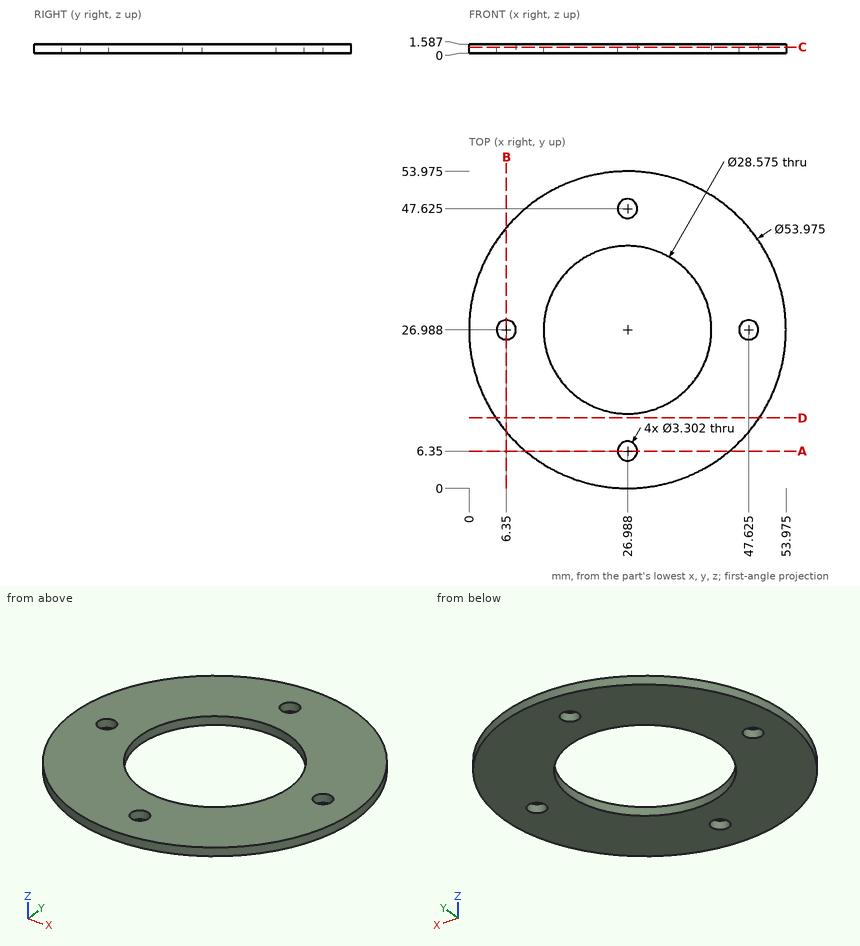
Job drawing, mm, ordinate dimensions from the low corner. One solid piece. Give positions to 0.01 mm unless a question says otherwise; leave off trailing zeros. Order: outer loops, then holes, each group sorted by start corner. A loop starts at its lowest first (then second) coordinate and runs counter-clockwise, first axis right, second up. Notation, with made-up numbers: (8.5, 80) - (62.5, 80) arc R26 ccw to (62.5, 116) - close; hole circle Ø9 at (56, 87.25). An arc over 180 degrees is marked (long way). Answer in a Markdown table with one row per item.
1. Saw through at C-C, the plane z = 1.05. Count the separate pieces of the cut face and the enclosed holes in it, plus the area to 3 significant figures.
Data:
| item | result |
|---|---|
| separate pieces | 1 |
| enclosed holes | 5 |
| area | 1,610 mm² |
2. Saw through at A-A, the plane y = 6.35. Give the cut face in (x, z).
Data:
| item | result |
|---|---|
| outline | (9.6, 0) - (25.34, 0) - (25.34, 1.59) - (9.6, 1.59) - close; (28.64, 0) - (44.38, 0) - (44.38, 1.59) - (28.64, 1.59) - close |
3. Probe probe 1 along X at (y, z) = (30.5, 0.55) (1 decimal); probe 2 along Y at (x, z) = (7, 0.55) (1 decimal); probe 3 along Y at (x, z) = (29, 0.5) (1 decimal). List the from-to ranges inside material, lowest first. Write a range as [from, to].
Data:
| item | result |
|---|---|
| probe 1 | x = [0.2, 13.1], [40.8, 53.7] |
| probe 2 | y = [8.9, 25.5], [28.5, 45.1] |
| probe 3 | y = [0.1, 12.8], [41.1, 53.9] |
4. Saw through at D-D, the plane y = 12. Give the cut face in (x, z) (1 decimal).
Data:
| item | result |
|---|---|
| outline | (4.5, 0) - (49.4, 0) - (49.4, 1.6) - (4.5, 1.6) - close |
